from build123d import *

# Parameters (mm, degrees)
F0_W     = 35
F0_H     = 60
F1_DEPTH = 15
F3_DEPTH = 25


with BuildPart() as f1:
    # F0 (on Top) → F1 (new body)
    with BuildSketch(Plane.XY):
        with Locations((17.5, 30)):
            Rectangle(F0_W, F0_H)
    extrude(amount=F1_DEPTH)

    # F2 (on face) → F3 (cut)
    with BuildSketch(Plane.XY.offset(15)):
        Polygon((23.9983939247, 10), (28.0146222424, 22.360679775), (17.5, 30), (6.9853777576, 22.360679775), (11.0016060753, 10), align=None)
    extrude(amount=-F3_DEPTH, mode=Mode.SUBTRACT)

    # F5 (on mid) → F6 (revolve)
    with BuildSketch(Plane.YZ.offset(17.5)):
        with BuildLine():
            Line((34.2611013353, 15), (39.2611013353, 15))
            ThreePointArc((39.2611013353, 15), (36.7611013353, 17.5), (34.2611013353, 15))
        make_face()
        with BuildLine():
            ThreePointArc((34.2611013353, 15), (36.7611013353, 12.5), (39.2611013353, 15))
            Line((39.2611013353, 15), (34.2611013353, 15))
        make_face()
    revolve(axis=Axis((17.5, 45.8512790501, 18.8291036189), (0, 0, 1)))


solid = f1.part
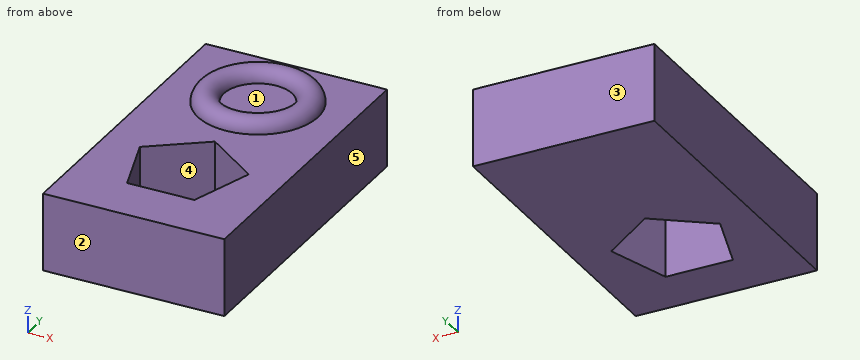
Design review of the part built by this model. Coordinates are the model's own, in mm. Face numbers are marked on the shaded views. A direction names the side the tool comes from. Round coordinates to 2 decimals unless told otherwise and drop trailing zeros. Write each loop counter-clockwise with the first axis right and the second up, starting at its lowest first coordinate (ties: lowest second). Pieces come first, ordered by that corner, then holes. Notation, with made-up numbers: (-9.5, 6.5) -> (0.5, 6.5) arc R13 cw to (0.5, 14.5) -> close; hole circle Ø5 at (61, 42). An arc over 180 degrees is marked (long way). One line per item, written item: value. Start each with the question number.
Q1. Add section A-A (z = 14.25). Give the boundary of the cut face in (x, y), then the cut area to 3 significant figures.
Q2. Add section C-C (x = 4). Give the boundary of the cut face in (y, z), then the cut area to 3 significant figures.
Q3. Insertion check: P1, Ø6.5, axis at x = 15, y = 46, coming from the +Z side. The pin has a flat end and moves straight along its axis. Give the tip position at first contact, or say it passes through.
Q4. Add section B-B (y = 27.5). Give the boundary of the cut face in (x, z), then the cut area to 3 significant figures.
Q5. Add section D-D (y = 18). Give the boundary of the cut face in (x, z).
Q6. Tool access review of the marked faces 4 and 5: name each direction out of +Z, -Z, +X, -X, +Y, -Y from which nothing blocks a thin tool from reaching the whole face with its end or side.
Q7. The part is to be moulded in two halves that separate along Y. For the marked faces 1, 2 and 3, say which applies: pulls with the +Y half, pulls with the -Y half, needs draft (parallel to the pull), parting line crosses it, or undercut.
Q8. To check wall thickness, follow probe 1 along Z at (x, y) = (8, 24); probe 2 along Y at (x, z) = (21.5, 16.5); probe 3 along Y at (x, z) = (12.5, 7.5). State the ranges of each line that lie inside material, in increasing order.
Response:
1. outline: (0, 0) -> (35, 0) -> (35, 60) -> (0, 60) -> close; hole (6.99, 22.36) -> (11, 10) -> (24, 10) -> (28.01, 22.36) -> (17.5, 30) -> close
1. area: 1,810 mm^2
2. outline: (0, 0) -> (60, 0) -> (60, 15) -> (0, 15) -> close
2. area: 900 mm^2
3. P1: stops at z = 15
4. outline: (0, 0) -> (14.06, 0) -> (14.06, 15) -> (0, 15) -> close; (20.94, 0) -> (35, 0) -> (35, 15) -> (20.94, 15) -> close
4. area: 422 mm^2
5. outline: (0, 0) -> (8.4, 0) -> (8.4, 15) -> (0, 15) -> close; (26.6, 0) -> (35, 0) -> (35, 15) -> (26.6, 15) -> close
6. face 4: +Z, -Z
6. face 5: +Z, -Z, +X, +Y, -Y
7. face 1: undercut
7. face 2: pulls with the -Y half
7. face 3: pulls with the +Y half
8. probe 1: z = 0 to 15
8. probe 2: y = 35.51 to 40, 51.71 to 56.19
8. probe 3: y = 0 to 10, 26.37 to 60
